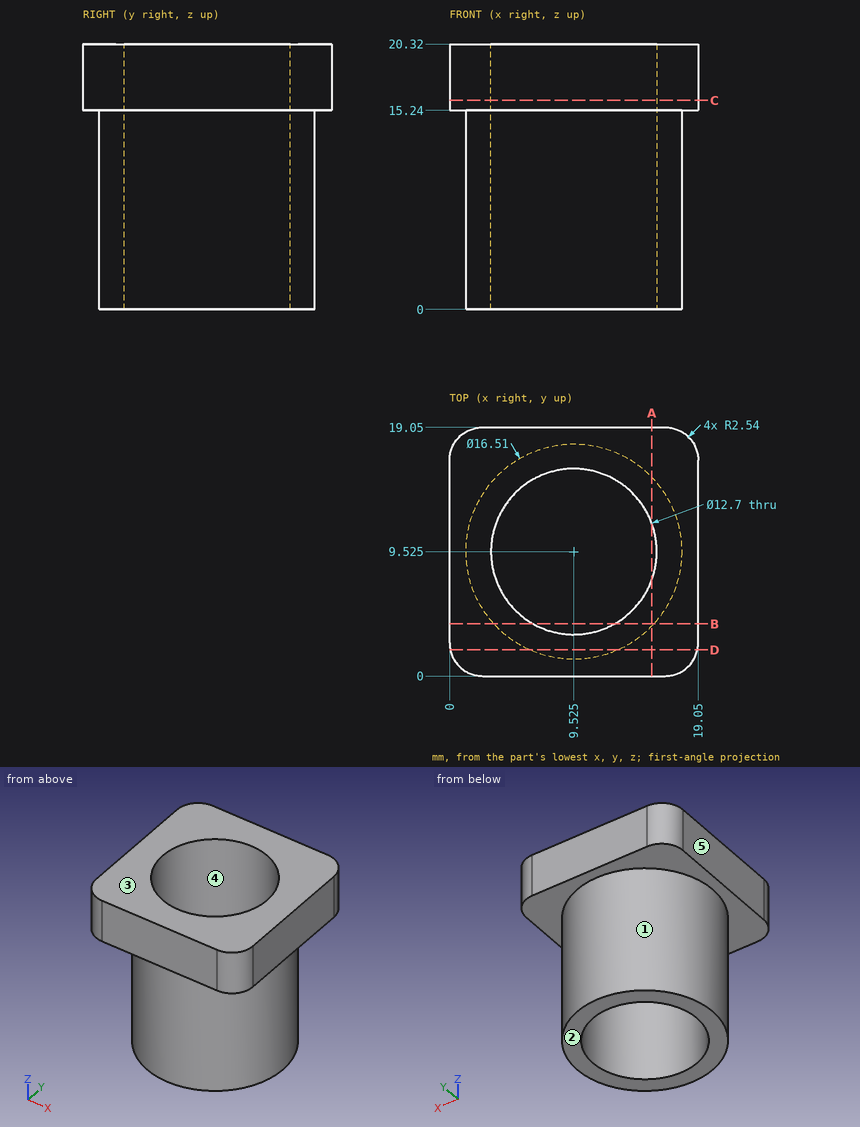
Print and shaded views of the part. All mm, measured from the part's lowest x, y and z. A direction names the side the tool comes from. Coordinates: 2 decimals unless noted, no trailing zeros. Order: outer loops, then holes, each group sorted by start corner. A loop starts at its lowest first (then second) coordinate and runs counter-clockwise, first axis right, second up. Notation, with made-up numbers: (6, 1) -> (45, 1) arc R19 cw to (45, 9) -> close; hole circle Ø9 at (40, 0.25). An arc over 180 degrees is marked (long way). Answer as a JSON object with one key per item and string values. Group by question number.
1) Cut at A-A, the plane x = 15.5. Write the cut outline in (y, z), then the cut area to 3 significant figures.
2) Cut at D-D, the plane y = 2. Write the cut outline in (x, z), then the cut area to 3 significant figures.
3) Which spindle directions (+Z, -Z, +X, -X, +Y, -Y) get a long thin tool onto all of the face, cutting with end or side? Do the marked faces 1 and 2. Say none if no direction does.
4) Flat gauge pins, fed straight in: pin 1 (4 mm diameter, centred on x = 12.5, y = 9, fed in from +Z); pin 2 (3 mm diameter, centred on x = 6.5, z = 6.5, fed in from +Y); pin 3 (2 mm diameter, centred on x = 4.5, z = 4, fed in from -Y); pin 4 (2 mm diameter, centred on y = 3.5, z = 7.5, fed in from -X). Where does each tip first touch, or does it go through?
5) Cut at C-C, the plane z = 16. Write the cut outline in (x, y) (3 decimals).
6) Cut at B-B, the plane y = 4. Write the cut outline in (x, z) (3 decimals), then the cut area to 3 significant figures.
7) Drill centre lines: L1, parallel to X at y = 9.25, z = 15; L2, parallel to X at y = 13.75, z = 17.5; L3, parallel to Z at x = 17.5, y = 4. Where is each one in solid material? Low to high.
8) Pull direction X, two halves, no side cores. Call the marked faces 3, 4 and 5: +X half, -X half, draft (parallel to the pull), parting line (faces both ways), or undercut.
Check values:
{
 "1": {"outline": "(0, 15.24) -> (3.83, 15.24) -> (3.83, 0) -> (7.38, 0) -> (7.38, 20.32) -> (0, 20.32) -> close; (11.67, 0) -> (15.22, 0) -> (15.22, 15.24) -> (19.05, 15.24) -> (19.05, 20.32) -> (11.67, 20.32) -> close", "area": "183 mm²"},
 "2": {"outline": "(0.06, 15.24) -> (6.13, 15.24) -> (6.13, 0) -> (12.92, 0) -> (12.92, 15.24) -> (18.99, 15.24) -> (18.99, 20.32) -> (0.06, 20.32) -> close", "area": "200 mm²"},
 "3": {"face 1": "-Z", "face 2": "-Z, +X, -X, +Y, -Y"},
 "4": {"pin 1": "passes through", "pin 2": "stops at y = 17.64", "pin 3": "stops at y = 2.32", "pin 4": "stops at x = 2.98"},
 "5": {"outline": "(0, 2.54) arc R2.54 ccw to (2.54, 0) -> (16.51, 0) arc R2.54 ccw to (19.05, 2.54) -> (19.05, 16.51) arc R2.54 ccw to (16.51, 19.05) -> (2.54, 19.05) arc R2.54 ccw to (0, 16.51) -> close; hole circle Ø12.7 at (9.525, 9.525)"},
 "6": {"outline": "(0, 15.24) -> (3.392, 15.24) -> (3.392, 0) -> (6.395, 0) -> (6.395, 20.32) -> (0, 20.32) -> close; (12.655, 0) -> (15.658, 0) -> (15.658, 15.24) -> (19.05, 15.24) -> (19.05, 20.32) -> (12.655, 20.32) -> close", "area": "157 mm²"},
 "7": {"L1": "x = 1.27 to 3.18, 15.87 to 17.78", "L2": "x = 0 to 4.78, 14.27 to 19.05", "L3": "z = 15.24 to 20.32"},
 "8": {"face 3": "draft", "face 4": "undercut", "face 5": "-X half"}
}
